Design review of the part built by this model. Coordinates are the model's own, in mm. Face numbers are marked on the shaded views. A direction names the side the tool comes from. Give positions to 0.01 mm unless a question says otherwise; leave off trailing zeros. Write each loop counter-clockwise with the first axis right and the second up, starting at its lowest first coordinate (ties: lowest second). Pieces come first, ordered by that corner, then holes. Notation, with made-up numbers: M 68.5,16 L 73.5,16 A17 ccw 73.5,30 Z; hole C 28,53 d4. An arc over 180 degrees is marked long. Answer in a Markdown table with one row per item.
```python
from build123d import *

# Parameters (mm, degrees)
SKETCH3_R           = 20
BOSS_EXTRUDE4_DEPTH = 400
SKETCH13_R          = 30
BOSS_EXTRUDE5_DEPTH = 20
BOSS_EXTRUDE6_START = 20
SKETCH14_R          = 30
BOSS_EXTRUDE6_DEPTH = 20
BOSS_EXTRUDE7_START = 50
SKETCH15_R          = 20
BOSS_EXTRUDE7_DEPTH = 50


with BuildPart() as part:
    # Sketch3 → Boss-Extrude4 (new body)
    with BuildSketch(Plane(origin=(0, 0, 0), x_dir=(1, 0, 0), z_dir=(0, 1, 0))):
        with Locations(Location((0, 0, 0), (0, 0, 270))):
            Circle(SKETCH3_R)
    extrude(amount=BOSS_EXTRUDE4_DEPTH)

    # Sketch13 → Boss-Extrude5 (add)
    with BuildSketch(Plane(origin=(0, 400, 0), x_dir=(1, 0, 0), z_dir=(0, 1, 0))):
        with Locations(Location((0, 0, 0), (0, 0, 270))):
            Circle(SKETCH13_R)
    extrude(amount=BOSS_EXTRUDE5_DEPTH)

    # Sketch14 → Boss-Extrude6 (add)
    with BuildSketch(Plane.XZ.offset(BOSS_EXTRUDE6_START)):
        with Locations(Location((0, 0, 0), (0, 0, 90))):
            Circle(SKETCH14_R)
    extrude(amount=-BOSS_EXTRUDE6_DEPTH)

    # Sketch15 → Boss-Extrude7 (add)
    with BuildSketch(Plane.XZ.offset(20).offset(BOSS_EXTRUDE7_START)):
        with Locations(Location((0, 0, 0), (0, 0, 90))):
            Circle(SKETCH15_R)
    extrude(amount=-BOSS_EXTRUDE7_DEPTH)


solid = part.part
```
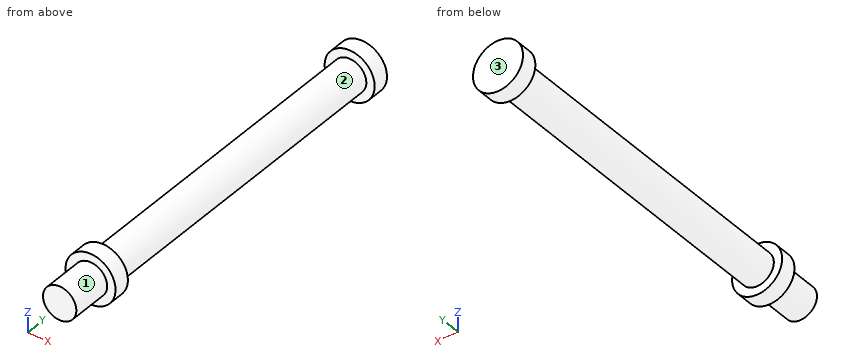
1) Add section C-C (x = 25). Write out the cut boundary in (y, z).
Geometry says:
| item | result |
|---|---|
| outline | M -20,-16.58 L 0,-16.58 L 0,16.58 L -20,16.58 Z; M 400,-16.58 L 420,-16.58 L 420,16.58 L 400,16.58 Z |
2) Add section B-B (z = 0). Write out the cut boundary in (x, y), and give its area (3 significant figures).
Geometry says:
| item | result |
|---|---|
| outline | M -30,-20 L -20,-20 L -20,-70 L 20,-70 L 20,-20 L 30,-20 L 30,0 L 20,0 L 20,400 L 30,400 L 30,420 L -30,420 L -30,400 L -20,400 L -20,0 L -30,0 Z |
| area | 20,400 mm^2 |
3) To check wall thickness, follow probe 1 along Y at (x, z) = (23.5, 15); probe 2 along X at (y, z) = (171.5, 1); probe 3 along X at (y, z) = (33.5, -11). State the ranges of each line that lie inside material, in increasing order. Write a range as [from, to].
Geometry says:
| item | result |
|---|---|
| probe 1 | [-20, 0], [400, 420] |
| probe 2 | [-19.97, 19.97] |
| probe 3 | [-16.7, 16.7] |
4) Insertion check: P1, Ø5, axis at x = 0, y = 18.5, coming from the +Z side; P2, Ø10, axis at y = 56, z = -7, coming from the -X side; P3, Ø1.5, axis at x = -8, y = 205.5, coming from the +Z side. Each pin has a flat end and moves straight along its axis. Give the tip position at first contact, or say it passes through.
Geometry says:
| item | result |
|---|---|
| P1 | z = 20 |
| P2 | x = -19.9 |
| P3 | z = 18.64 |
5) Add section A-A (x = 0). Write out the cut boundary in (y, z).
Geometry says:
| item | result |
|---|---|
| outline | M -70,-20 L -20,-20 L -20,-30 L 0,-30 L 0,-20 L 400,-20 L 400,-30 L 420,-30 L 420,30 L 400,30 L 400,20 L 0,20 L 0,30 L -20,30 L -20,20 L -70,20 Z |
6) For the marked faces 1, 2 and 3, list the 3-axis set-ups (+Z, -Z, +X, -X, +Y, -Y) from which the entire face can be reached by the end or side of a thin tool; tool diameter is ignored.
Geometry says:
| item | result |
|---|---|
| face 1 | -Y |
| face 2 | none |
| face 3 | +Z, -Z, +X, -X, +Y |
7) Add section D-D (y = 288). Write out the cut boundary in (x, z), and give its area (3 significant figures).
Geometry says:
| item | result |
|---|---|
| outline | C 0,0 d40 |
| area | 1,260 mm^2 |
